Geometry check sheet. Reference: the model listing, model coordinates, mm. A direction names the side the tool comes from. Give positions to 0.01 mm unless a question says otherwise; leave off trailing zeros. Loops run counter-clockwise (first coordinate to the right, second up) from the corner with the lowest first, then second, coordinate; pieces in that order, holes last.
```python
from build123d import *

# Parameters (mm, degrees)
F1_DEPTH = 10
F2_DEPTH = 30.7
F3_DEPTH = 20
F4_R     = 11
F4_R_2   = 2.5
F5_DEPTH = 2
F6_DEPTH = 26
F8_DEPTH = 19.2
F4_R_3   = 1.5
F9_DEPTH = 4.5


with BuildPart() as f1:
    # F0 (on Front) → F1 (new body)
    with BuildSketch(Plane.XZ):
        Polygon((-21.15, 11.15), (-11.15, 21.15), (-16.15, 21.15), (-21.15, 16.15), align=None)
        Polygon((-11.15, -21.15), (-21.15, -11.15), (-21.15, -16.15), (-16.15, -21.15), align=None)
        Polygon((21.15, -16.15), (21.15, -11.15), (11.15, -21.15), (16.15, -21.15), align=None)
        Polygon((16.15, 21.15), (11.15, 21.15), (21.15, 11.15), (21.15, 16.15), align=None)
        Polygon((11.15, 21.15), (-11.15, 21.15), (-21.15, 11.15), (-21.15, -11.15), (-11.15, -21.15), (-8, -21.15), (8, -21.15), (11.15, -21.15), (21.15, -11.15), (21.15, 11.15), align=None)
    extrude(amount=F1_DEPTH)

    # F0 (on Front) → F2 (join)
    with BuildSketch(Plane.XZ):
        Polygon((11.15, 21.15), (-11.15, 21.15), (-21.15, 11.15), (-21.15, -11.15), (-11.15, -21.15), (-8, -21.15), (8, -21.15), (11.15, -21.15), (21.15, -11.15), (21.15, 11.15), align=None)
        Polygon((-21.15, 11.15), (-11.15, 21.15), (-16.15, 21.15), (-21.15, 16.15), align=None)
        Polygon((16.15, 21.15), (11.15, 21.15), (21.15, 11.15), (21.15, 16.15), align=None)
        Polygon((-11.15, -21.15), (-21.15, -11.15), (-21.15, -16.15), (-16.15, -21.15), align=None)
        Polygon((21.15, -16.15), (21.15, -11.15), (11.15, -21.15), (16.15, -21.15), align=None)
        Polygon((8, -21.15), (-8, -21.15), (-8, -31.15), (0, -31.15), (8, -31.15), align=None)
    extrude(amount=-F2_DEPTH)

    # F0 (on Front) → F3 (cut)
    with BuildSketch(Plane.XZ):
        Polygon((16.15, 21.15), (11.15, 21.15), (21.15, 11.15), (21.15, 16.15), align=None)
        Polygon((-21.15, 11.15), (-11.15, 21.15), (-16.15, 21.15), (-21.15, 16.15), align=None)
        Polygon((-11.15, -21.15), (-21.15, -11.15), (-21.15, -16.15), (-16.15, -21.15), align=None)
        Polygon((21.15, -16.15), (21.15, -11.15), (11.15, -21.15), (16.15, -21.15), align=None)
        Polygon((8, -21.15), (-8, -21.15), (-8, -31.15), (0, -31.15), (8, -31.15), align=None)
    extrude(amount=-F3_DEPTH, mode=Mode.SUBTRACT)

    # F4 (on face) → F5 (join)
    with BuildSketch(Plane.XZ.offset(10)):
        Circle(F4_R)
        Circle(F4_R_2, mode=Mode.SUBTRACT)
    extrude(amount=F5_DEPTH)

    # F4 (on face) → F6 (join)
    with BuildSketch(Plane.XZ.offset(10)):
        Circle(F4_R_2)
    extrude(amount=F6_DEPTH)

    # F7 (on face) → F8 (cut)
    with BuildSketch(Plane.XZ.offset(36)):
        with BuildLine():
            Line((1.5, -2), (-1.5, -2))
            ThreePointArc((-1.5, -2), (0, -2.5), (1.5, -2))
        make_face()
    extrude(amount=-F8_DEPTH, mode=Mode.SUBTRACT)

    # F4 (on face) → F9 (cut)
    with BuildSketch(Plane.XZ.offset(10)):
        with Locations((-15.5, 15.5)):
            Circle(F4_R_3)
        with Locations((15.5, 15.5)):
            Circle(F4_R_3)
        with Locations((15.5, -15.5)):
            Circle(F4_R_3)
        with Locations((-15.5, -15.5)):
            Circle(F4_R_3)
    extrude(amount=-F9_DEPTH, mode=Mode.SUBTRACT)


solid = f1.part
```
1) Scan lines: line 1 along Z through (x, y) = (15.5, -7.4); line 2 along X through (y, z) = (-8, -15); line 3 along Y through (x, z) = (-1, -9). Record each from-to range of solid material in increasing order.
2) Mould release check, pull along Y, two halves, no side actions. Record for faces 1 (the flat face through (0, 20, -26)), 2 (the flat face through (17, 20, 17)), 3 (the flat face through (21.15, 10, 0)): +Y half, -Y half, draft (parallel to the pull), parting line (faces both ways), or undercut.
3) Sectioned sample at B-B on x = 0. Enter the section's corners in (y, z).
4) Tool access check on faces 4 (the flat face through (-16.2, 9.9, 16.1)), 5 (the cylindrical face through (-17, -7.78, 15.57)), 6 (the flat face through (17, 0, 17)). Record the directions out of +Z, -Z, +X, -X, +Y, -Y that give a thin tool (end or side, any length) a straight path to the whole face; none if there is none.
5) Sectioned sample at C-C on z = 18. Enter the section's corners in (x, y), plus the area to 3 significant figures.
6) Sectioned sample at D-D on y = 10.5. Enter the section's corners in (x, z), plus the area to 3 significant figures.
7) Sectioned sample at A-A on y = 25.5. Enter the section's corners in (x, z).
8) Depth check by flat-ended pin: P1, Ø8, axis at y = -14.5, z = -5.5, coming from the +X side; P2, Ø1.5, axis at x = -15, z = 15, coming from the -Y side; P3, Ø11, axis at y = 23.5, z = -27.5, coming from the -X side. Enter the tip coordinate at first touch or a pass-through.
Determined:
1. line 1: z = -21.15 to -17, -14 to 14, 17 to 21.15
1. line 2: x = -21.15 to -16.91, -14.09 to 14.09, 16.91 to 21.15
1. line 3: y = -12 to 30.7
2. face 1: -Y half
2. face 2: undercut
2. face 3: draft
3. outline: (-36, -2) - (-16.8, -2) - (-16.8, -2.5) - (-12, -2.5) - (-12, -11) - (-10, -11) - (-10, -21.15) - (20, -21.15) - (20, -31.15) - (30.7, -31.15) - (30.7, 21.15) - (-10, 21.15) - (-10, 11) - (-12, 11) - (-12, 2.5) - (-36, 2.5) - close
4. face 4: +Z, -X
4. face 5: -Y
4. face 6: +Z, +X
5. outline: (-19.3, -10) - (19.3, -10) - (19.3, 0) - (14.3, 0) - (14.3, 20) - (19.3, 20) - (19.3, 30.7) - (-19.3, 30.7) - (-19.3, 20) - (-14.3, 20) - (-14.3, 0) - (-19.3, 0) - close
5. area: 1,370 mm2
6. outline: (-21.15, -11.15) - (-11.15, -21.15) - (11.15, -21.15) - (21.15, -11.15) - (21.15, 11.15) - (11.15, 21.15) - (-11.15, 21.15) - (-21.15, 11.15) - close
6. area: 1,590 mm2
7. outline: (-21.15, -16.15) - (-16.15, -21.15) - (-8, -21.15) - (-8, -31.15) - (8, -31.15) - (8, -21.15) - (16.15, -21.15) - (21.15, -16.15) - (21.15, 16.15) - (16.15, 21.15) - (-16.15, 21.15) - (-21.15, 16.15) - close
8. P1: stops at x = 10.74
8. P2: stops at y = -5.5
8. P3: stops at x = -8
